Can you work these out from the model? Positions are in its coordinate system, mm. Coordinates: 2 decimals unless noted, no trailing zeros. Order: outer loops, then holes, each group sorted by start corner. A loop starts at its lowest first (then second) coordinate and runs counter-clockwise, first axis right, second up. Notation, with made-up numbers: (-35, 26) -> (-28, 26) arc R26 cw to (-28, 49) -> close; hole circle Ø4 at (7, 48.5). An arc over 180 degrees is marked (long way). Answer in a Markdown table with one row per item.
Autodesk Inventor part; units mm, degrees
ref_plane "YZ Plane" through (0, 0, 0) normal (1, 0, 0) x (0, 1, 0)
ref_plane "XZ Plane" through (0, 0, 0) normal (0, 1, 0) x (-1, 0, 0)
ref_plane "XY Plane" through (0, 0, 0) normal (0, 0, 1) x (1, 0, 0)
sketch "Sketch1" plane through (0, 0, 0) normal (0, 0, 1) x (1, 0, 0)
  line L0 (0, 0) -> (9, 0)
  line L1 (9, 0) -> (9, 59)
  line L2 (9, 59) -> (0, 59)
  line L3 (0, 59) -> (0, 0)
  circle A0 centre (4.5, 55.75) radius 1.5
  circle A1 centre (4.5, 3.25) radius 1.5
  line L4 (4.5, 55.75) -> (4.5, 3.25) construction
  circle A2 centre (4.5, 29.5) radius 1.5
  point P0 (9, 29.5)
  point P1 (4.5, 59)
  dimension "d0" = 9
  dimension "d1" = 59
  dimension "d2" = 3
  dimension "d3" = 3
  dimension "d4" = 52.5
  dimension "d5" = 3
extrude "Extrusion1" add sketch "Sketch1" along normal blind 5
properties part number "SJ017" material "ABS Plastic"
(1) Suppose I cut it at B-B (x = 4.5). Please give me the cut outline in (y, z), and give its area (3 significant figures).
Response values:
| item | result |
|---|---|
| outline | (0, 0) -> (1.75, 0) -> (1.75, 5) -> (0, 5) -> close; (4.75, 0) -> (28, 0) -> (28, 5) -> (4.75, 5) -> close; (31, 0) -> (54.25, 0) -> (54.25, 5) -> (31, 5) -> close; (57.25, 0) -> (59, 0) -> (59, 5) -> (57.25, 5) -> close |
| area | 250 mm2 |
(2) We'd pull the mould along Y, two halves only. Please class faces 1 (the flat face through (4, 0, 2)), 2 (the cylindrical face through (4.305, 28.013, 2.465)), 3 (the flat face through (9, 29, 2)): +Y half, -Y half, draft (parallel to the pull), parting line (faces both ways), or undercut.
Response values:
| item | result |
|---|---|
| face 1 | -Y half |
| face 2 | undercut |
| face 3 | draft |
(3) Will this pin go through, and if not, where does the flat tip stop? pin 1 Ø1.8 at (x, y) = (4.5, 55.75) entering from -Z.
Response values:
| item | result |
|---|---|
| pin 1 | through |
(4) I need wall thicknesses on line 1 (Y direction, x = 4.5, z = 1.8); line 2 (Y direction, x = 4, z = 0.85). Which ranges of each line are inside material? Lowest first, please. Write a range as [from, to].
Response values:
| item | result |
|---|---|
| line 1 | [0, 1.75], [4.75, 28], [31, 54.25], [57.25, 59] |
| line 2 | [0, 1.84], [4.66, 28.09], [30.91, 54.34], [57.16, 59] |
(5) Suppose I cut it at C-C (z = 3.25). Please give me the cut outline in (x, y).
Response values:
| item | result |
|---|---|
| outline | (0, 0) -> (9, 0) -> (9, 59) -> (0, 59) -> close; hole circle Ø3 at (4.5, 3.25); hole circle Ø3 at (4.5, 29.5); hole circle Ø3 at (4.5, 55.75) |
(6) Suppose I cut it at A-A (y = 29.5). Please give me the cut outline in (x, z), and give its area (3 significant figures).
Response values:
| item | result |
|---|---|
| outline | (0, 0) -> (3, 0) -> (3, 5) -> (0, 5) -> close; (6, 0) -> (9, 0) -> (9, 5) -> (6, 5) -> close |
| area | 30.0 mm2 |
